```python
from build123d import *

# Parameters (mm, degrees)
ESBO_O1_R                = 1.6
ESBO_O1_W                = 10
ESBO_O1_H                = 3
RESSALTO_EXTRUS_O1_DEPTH = 3
FILETE1_R                = 5
FILETE3_R                = 3
FILETE4_R                = 10
FILETE2_R                = 5


with BuildPart() as part:
    # Esboço1 → Ressalto-extrusão1 (new body)
    with BuildSketch(Plane.XY):
        with BuildLine():
            Line((-0.781024968, 23), (-31.296028058, 23))
            Line((-31.296028058, 23), (-41.498532893, 30))
            Line((-41.498532893, 30), (-56.498532893, 30))
            Line((-56.498532893, 30), (-66.701037728, 23))
            Line((-66.701037728, 23), (-80.742879141, -37.388961655))
            Line((-80.742879141, -37.388961655), (-65.645638728, -40.899422008))
            Line((-65.645638728, -40.899422008), (-66.494943652, -44.551980173))
            Line((-66.494943652, -44.551980173), (-56.754788546, -46.816793304))
            Line((-56.754788546, -46.816793304), (-55.905483622, -43.164235139))
            Line((-55.905483622, -43.164235139), (-40.808243208, -46.674695492))
            Line((-40.808243208, -46.674695492), (-29.955288394, 0))
            Line((-29.955288394, 0), (10, 0))
            Line((10, 0), (10, 23))
            Line((10, 23), (0.781024968, 23))
            ThreePointArc((0.781024968, 23), (0, 16.9), (-0.781024968, 23))
        make_face()
        with Locations((-60.492459533, -40.814309185)):
            Circle(ESBO_O1_R, mode=Mode.SUBTRACT)
        Polygon((-34.444555902, -6.06061562), (-38.974182165, -25.540925831), (-41.896228696, -24.861481892), (-37.366602434, -5.381171681), align=None, mode=Mode.SUBTRACT)
        Polygon((-70.142678503, -18.293523812), (-73.064725034, -17.614079872), (-68.535098772, 1.866230339), (-65.61305224, 1.1867864), align=None, mode=Mode.SUBTRACT)
        Polygon((-53.868610446, 9.749384541), (-50.787533444, 23), (-41.047378339, 20.735186869), (-44.12845534, 7.48457141), (-38.771370032, 6.238924188), (-48.283585183, -34.669727256), (-68.737910905, -29.91361968), (-59.225695754, 10.995031763), align=None, mode=Mode.SUBTRACT)
        with Locations((-60.676910422, 18)):
            Circle(ESBO_O1_R, mode=Mode.SUBTRACT)
        with Locations((0, 4.5)):
            Rectangle(ESBO_O1_W, ESBO_O1_H, mode=Mode.SUBTRACT)
        with Locations((-23, 11)):
            Circle(ESBO_O1_R, mode=Mode.SUBTRACT)
        with Locations((-20, 18.5)):
            Rectangle(ESBO_O1_W, ESBO_O1_H, mode=Mode.SUBTRACT)
        with Locations((5, 11)):
            Circle(ESBO_O1_R, mode=Mode.SUBTRACT)
    extrude(amount=RESSALTO_EXTRUS_O1_DEPTH)

    # Filete1
    filete1_edges = [part.edges().sort_by_distance(p)[0] for p in [
        (10, 0, 1.5),
        (-40.808243208, -46.674695492, 1.5),
        (-80.742879141, -37.388961655, 1.5),
    ]]
    fillet(filete1_edges, radius=FILETE1_R)

    # Filete3
    filete3_edges = [part.edges().sort_by_distance(p)[0] for p in [
        (10, 23, 1.5),
        (-55.905483622, -43.164235139, 1.5),
        (-65.645638728, -40.899422008, 1.5),
        (-53.868610446, 9.749384541, 1.5),
        (-44.12845534, 7.48457141, 1.5),
        (-41.047378339, 20.735186869, 1.5),
        (-50.787533444, 23, 1.5),
    ]]
    fillet(filete3_edges, radius=FILETE3_R)

    # Filete4
    filete4_edges = [part.edges().sort_by_distance(p)[0] for p in [
        (-29.955288394, 0, 1.5),
    ]]
    fillet(filete4_edges, radius=FILETE4_R)

    # Filete2
    filete2_edges = [part.edges().sort_by_distance(p)[0] for p in [
        (-56.754788546, -46.816793304, 1.5),
        (-66.494943652, -44.551980173, 1.5),
        (-31.296028058, 23, 1.5),
        (-41.498532893, 30, 1.5),
        (-56.498532893, 30, 1.5),
        (-66.701037728, 23, 1.5),
    ]]
    fillet(filete2_edges, radius=FILETE2_R)


solid = part.part
```
The listing builds one solid part. Answer for the finished solid, in the listing's coordinates (mm). A direction names the side the tool comes from. Round coordinates to 2 decimals unless told otherwise and drop trailing zeros. Order: outer loops, then holes, each group sorted by start corner. A loop starts at its lowest first (then second) coordinate and runs counter-clockwise, first axis right, second up. Notation, with made-up numbers: (48, -24) -> (56, -24) arc R21 ccw to (56, -1) -> close; hole circle Ø6 at (-24, -21.75). An arc over 180 degrees is marked (long way). Answer as CSV lines item,"result".
Q1. A cutting plane is placed at B-B on y = -23. Determine the outline of the cut face in (x, z), plus the area to 3 significant figures.
Computed values:
outline,"(-77.4, 0) -> (-67.13, 0) -> (-67.13, 3) -> (-77.4, 3) -> close; (-45.57, 0) -> (-41.46, 0) -> (-41.46, 3) -> (-45.57, 3) -> close; (-38.38, 0) -> (-35.3, 0) -> (-35.3, 3) -> (-38.38, 3) -> close"
area,"52.4 mm^2"
Q2. Consider line 1 (Y direction, x = 0, z = 0.95); line 2 (X direction, y = 10, z = 0.45); line 3 (Y direction, x = -21, z = 1.25). Determine where each line is inside the solid, lowest interval first. Write a range as from..to.
Computed values:
line 1,"y = 0..3, 6..16.9"
line 2,"x = -69.72..-59.46, -43.51..-24.25, -21.75..3.75, 6.25..10"
line 3,"y = 0..17, 20..23"
Q3. A cutting plane is placed at C-C on y = -12. Determine the outline of the cut face in (x, z).
Computed values:
outline,"(-74.84, 0) -> (-71.76, 0) -> (-71.76, 3) -> (-74.84, 3) -> close; (-68.68, 0) -> (-64.57, 0) -> (-64.57, 3) -> (-68.68, 3) -> close; (-43.01, 0) -> (-38.91, 0) -> (-38.91, 3) -> (-43.01, 3) -> close; (-35.83, 0) -> (-32.75, 0) -> (-32.75, 3) -> (-35.83, 3) -> close"
Q4. A cutting plane is placed at A-A on x = -23. Determine the outline of the cut face in (y, z).
Computed values:
outline,"(-0.05, 0) -> (9.4, 0) -> (9.4, 3) -> (-0.05, 3) -> close; (12.6, 0) -> (17, 0) -> (17, 3) -> (12.6, 3) -> close; (20, 0) -> (23, 0) -> (23, 3) -> (20, 3) -> close"
Q5. Given pin 1 (1.5 mm diameter, centred on x = -22, z = 1.5, fed in from +Y); pin 2 (3 mm diameter, centred on x = -67, y = -17, fed in from -Z); pin 3 (1.5 mm diameter, centred on y = 5, z = 1.5, fed in from -X); pin 4 (1.5 mm diameter, centred on y = 18.5, z = 1, fed in from -X), each flat-ended and moving along its own axis, determine where each tip first touches the part or whether it passes through.
Computed values:
pin 1,"stops at y = 23"
pin 2,"stops at z = 0"
pin 3,"stops at x = -71.06"
pin 4,"stops at x = -67.92"
Q6. Which of the six approach directions +Z, -Z, +X, -X, +Y, -Y give full straight-line access (tool end or side, diameter ignored) to faces 1 (the flat face through (-64.05, -9.75, 1.48)), 2 (the flat face through (-15, 23, 1)), 3 (the flat face through (-49.38, -44.68, 1.48))?
Computed values:
face 1,"+Z, -Z"
face 2,"+Z, -Z, +X, +Y"
face 3,"+Z, -Z, -Y"
Q7. For a pull along X with two mould halves and no side action, classify faces 4 (the flat face through (-42.576, 14.162, 1.479)), 5 (the flat face through (-9, 0, 1)), 6 (the flat face through (-61.64, -45.68, 1.48)) as +X half, -X half, draft (parallel to the pull), parting line (faces both ways), or undercut.
Computed values:
face 4,"undercut"
face 5,"draft"
face 6,"-X half"
Q8. A cutting plane is placed at D-D on z = 2.2. Give the number of separate pieces and of enclosed holes in the cut face, plus the area to 3 significant figures.
Computed values:
separate pieces,"1"
enclosed holes,"9"
area,"2,540 mm^2"
